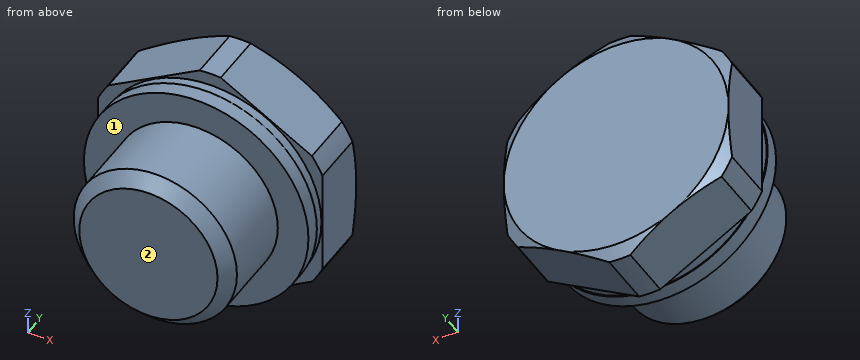
Solid Edge part; units mm, degrees
sketch "Sketch1" plane through (0, 0, 0) normal (0, 0, 1) x (1, 0, 0)
  line L0 (0, 17) -> (11, 17)
  line L1 (11, 17) -> (12.15, 16.336)
  line L2 (12.15, 16.336) -> (12.15, 11)
  line L3 (12.15, 11) -> (10.9, 11)
  line L4 (10.9, 11) -> (10.9, 10)
  line L5 (10.9, 10) -> (8, 10)
  line L6 (8, 10) -> (8, 1.227)
  line L7 (8, 1.227) -> (6.773, 0)
  line L8 (6.773, 0) -> (0, 0)
  line L9 (0, 0) -> (0, 17)
revolve "RevolvedProtrusion1" add sketch "Sketch1" angle 360 about axis through (0, 0, 0) along (0, 1, 0)
cosmetic_thread "Thread1"
sketch "Sketch2" plane through (0, 10, 0) normal (0, -1, 0) x (1, 0, 0)
  circle A0 centre (0, 0) radius 27
  line L0 (-11, 6.3509) -> (0, 12.7017)
  line L1 (0, 12.7017) -> (11, 6.3509)
  line L2 (11, 6.3509) -> (11, -6.3509)
  line L3 (11, -6.3509) -> (0, -12.7017)
  line L4 (0, -12.7017) -> (-11, -6.3509)
  line L5 (-11, -6.3509) -> (-11, 6.3509)
extrude "ExtrudedCutout_1" cut sketch "Sketch2" against normal blind 7
sketch "Sketch3" plane through (0, 0, 0) normal (0, 0, 1) x (1, 0, 0)
  line L0 (8, 8.5) -> (11, 8.5)
  line L1 (11, 8.5) -> (11, 10)
  line L2 (11, 10) -> (8, 10)
  line L3 (8, 10) -> (8, 8.5)
revolve "RevolvedProtrusion2" add sketch "Sketch3" angle 360 about axis through (0, 8.5, 0) along (0, 1, 0)
properties part number "28027-221615"
Build history of the part. All positions in model axes, mm. Face numbers are marked on the shaded views. A direction names the side the tool comes from. Give positions to 0.01 mm unless a question says otherwise; leave off trailing zeros. Loops run counter-clockwise (first coordinate to the right, second up) from the corner with the lowest first, then second, coordinate; pieces in that order, holes last. Notation, with made-up numbers: (50, 69) -> (100, 69) arc R3 cw to (100, 73) -> close; hole circle Ø6 at (24.5, 56). An arc over 180 degrees is marked (long way). One line per question, with ' | ' between items. Start each with the question number.
1) Pin check, flat tips, straight feed: pin 1 (4 mm diameter, centred on y = 2.5, z = 7.5, fed in from -X); pin 2 (1.5 mm diameter, centred on y = 14.5, z = -7.5, fed in from -X); pin 3 (4 mm diameter, centred on x = -7, y = 3.5, fed in from -Z) (3 decimals). Stop position of each tip, or through.
2) Cut at A-A (y = 12.25). Give the cut face in (x, z), plus the area to 3 significant figures.
3) Cut at C-C (y = 6). Give the cut face in (x, z), plus the area to 3 significant figures.
4) 3-axis set-ups, long thin cutter, end or side, ignore diameter. For the marked faces 1 and 2: which of +Z, -Z, +X, -X, +Y, -Y reach the whole face in a straight line?
5) Cut at B-B (x = 0). Give the cut face in (y, z), plus the area to 3 significant figures.
6) Probe L1, parallel to Y at x = 9.25, z = -3; L2, parallel to Z at x = -3.5, y = 16; L3, parallel to Z at x = 9, y = 12. List the from-to ranges inside material, lowest first.
Return value:
1) pin 1: x = -5.81 | pin 2: x = -10.1 | pin 3: z = -6.245
2) outline: (-11, -5.16) arc R12.15 ccw to (-9.97, -6.95) -> (-1.03, -12.11) arc R12.15 ccw to (1.03, -12.11) -> (9.97, -6.95) arc R12.15 ccw to (11, -5.16) -> (11, 5.16) arc R12.15 ccw to (9.97, 6.95) -> (1.03, 12.11) arc R12.15 ccw to (-1.03, 12.11) -> (-9.97, 6.95) arc R12.15 ccw to (-11, 5.16) -> close | area: 416 mm^2
3) outline: circle Ø16 at (0, 0) | area: 201 mm^2
4) face 1: -Y | face 2: +Z, -Z, +X, -X, -Y
5) outline: (0, -6.77) -> (1.23, -8) -> (8.5, -8) -> (8.5, -11) -> (10, -11) -> (10, -10.9) -> (11, -10.9) -> (11, -12.15) -> (16.34, -12.15) -> (17, -11) -> (17, 11) -> (16.34, 12.15) -> (11, 12.15) -> (11, 10.9) -> (10, 10.9) -> (10, 11) -> (8.5, 11) -> (8.5, 8) -> (1.23, 8) -> (0, 6.77) -> close | area: 334 mm^2
6) L1: 8.5 to 17 | L2: -10.68 to 10.68 | L3: -7.51 to 7.51
